from build123d import *

# Parameters (mm, degrees)
F0_W        = 20
F0_H        = 60
F1_DEPTH    = 150
F2_D        = 6
F2_DEPTH    = 50
F2_TIP      = 1.8025818571
F3_SIZE2    = 29.99999
F3_SIZE     = 149.99999
F3_2_SIZE2  = 29.99999
F3_2_SIZE   = 149.99999
F4_T1_DEPTH = 407.0708695577
F4_T3_DEPTH = 407.0708695577


# Not quite as in the source:
# - a fillet or chamfer that OpenCascade refuses, or shapes differently, is made with other operations: its cross-section is extruded or revolved along the edge and cut away or added
# - a fillet or chamfer is up to 0.001 mm smaller than in the source, because OpenCascade refuses the exact size


with BuildPart() as f1:
    # F0 (on Top) → F1 (new body)
    with BuildSketch(Plane.XY):
        Rectangle(F0_W, F0_H)
    extrude(amount=F1_DEPTH)

    # F2
    with Locations(Plane(origin=(0, 0, 0), x_dir=(1, 0, 0), z_dir=(0, 0, -1))):
        with Locations((0, -10), (0, 0), (0, 10)):
            Hole(F2_D / 2, depth=F2_DEPTH)
            with Locations((0, 0, -(F2_DEPTH + F2_TIP / 2))):  # 118° drill point
                Cone(0, F2_D / 2, F2_TIP, mode=Mode.SUBTRACT)

    # F3 (size 150 and 30 in the source; OpenCascade refuses exactly that, so slightly less here)
    f3_edges = [f1.edges().sort_by_distance(p)[0] for p in [
        (0, -30, 150),
    ]]
    f3_side = f1.faces().sort_by_distance((0, -30, 75))[0]
    chamfer(f3_edges, length=F3_SIZE, length2=F3_SIZE2, reference=f3_side)

    # F3#2 (size 150 and 30 in the source; OpenCascade refuses exactly that, so slightly less here)
    f3_2_edges = [f1.edges().sort_by_distance(p)[0] for p in [
        (0, 30, 150),
    ]]
    f3_2_side = f1.faces().sort_by_distance((0, 30, 75))[0]
    chamfer(f3_2_edges, length=F3_2_SIZE, length2=F3_2_SIZE2, reference=f3_2_side)

    # F4: chamfer of 24.5 x 10 on 4 edges, made by hand

    # F4_s2 → F4_t1 (cut)
    with BuildSketch(Plane(origin=(0, -38.5287100353, -192.6436015479), x_dir=(1, 0, 0), z_dir=(0, 0.1961160849, 0.9805806857))):
        Polygon((0, -29.4174225336), (10, -4.9174225336), (10, -29.4174225336), align=None)
        Polygon((-10, -4.9174225336), (0, -29.4174225336), (-10, -29.4174225336), align=None)
    extrude(amount=F4_T1_DEPTH, mode=Mode.SUBTRACT)

    # F4_s4 → F4_t3 (cut)
    with BuildSketch(Plane(origin=(0, 38.5287100353, -192.6436015479), x_dir=(1, 0, 0), z_dir=(0, -0.1961160849, 0.9805806857))):
        Polygon((0, 29.4174225336), (10, 4.9174225336), (10, 29.4174225336), align=None)
        Polygon((-10, 4.9174225336), (0, 29.4174225336), (-10, 29.4174225336), align=None)
    extrude(amount=F4_T3_DEPTH, mode=Mode.SUBTRACT)


solid = f1.part
Source: CAD feature listing. Evaluate the final solid. Frame: model axes, mm. A direction names the side the tool comes from. Give positions to 0.01 mm unless a question says otherwise; leave off trailing zeros. Write each loop counter-clockwise with the first axis right and the second up, starting at its lowest first coordinate (ties: lowest second). Pieces come first, ordered by that corner, then holes. Notation, with made-up numbers: M 85,-13.75 L 127,-13.75 A33 cw 127,24.25 Z; hole C 4,52.25 d9. An arc over 180 degrees is marked long. Return JSON: item names as keys, results as strings. Group by question number.
1) Pin query (flat end, axial travel): P1, Ø1.5, axis at y = 5, z = 83, coming from the +X side; P2, Ø4, axis at y = 8.5, z = 107, coming from the +X side; P3, Ø1.5, axis at y = -1.5, z = 47, coming from the +X side. Return the tip coordinate at first contact, or that it passes through.
2) Cut plane A-A, the plane z = 27.5. Output: boundary loops of the cut face in (x, y), plus the area to 3 significant figures.
3) Cut plane C-C, the plane x = 7.5. Output: boundary loops of the cut face in (y, z), plus the area to 3 significant figures.
4) Material intervals for line 1 along Y through (x, z) = (-1.5, 8); line 2 along X through (y, z) = (11, 19); line 3 along X through (y, z) = (10, 23.5), sorted ascending. Write a range as [from, to].
5) Pull-direction query (Y, two-part tool) for faces 1 (the face through (4, 0, 0)), 2 (the face through (-3.96, 9.03, 55.38)), 3 (the face through (0.24, 0.46, 51.49)), 4 (the face through (0.24, 10.46, 51.49)); classes: pulls with the +Y half, pulls with the -Y half, needs draft (parallel to the pull), parting line crosses it, or undercut.
6) Cut plane D-D, the plane z = 64.5. Output: boundary loops of the cut face in (x, y).
7) Set-up query: faces 5 (the face through (-10, 0, 10)), 6 (the face through (3, -10, 25)). Return all of +Z, -Z, +X, -X, +Y, -Y with unobstructed straight access to the full face (end or side cutting, diameter ignored); none if empty.
8) Cut plane B-B, the plane y = -15.5. Output: boundary loops of the cut face in (x, z), plus the area to 3 significant figures.
Recorded:
{
 "1": {"P1": "stops at x = 3.67", "P2": "stops at x = 0.86", "P3": "stops at x = 7.95"},
 "2": {"outline": "M -9.81,0 L 0,-24.5 L 9.81,0 L 0,24.5 Z; hole C 0,-10 d6; hole C 0,0 d6; hole C 0,10 d6", "area": "396 mm²"},
 "3": {"outline": "M -11.26,0 L 11.26,0 L 0,56.31 Z", "area": "634 mm²"},
 "4": {"line 1": "y = [-24.65, -12.6], [-7.4, -2.6], [2.6, 7.4], [12.6, 24.65]", "line 2": "x = [-6.08, -2.83], [2.83, 6.08]", "line 3": "x = [-6.12, -3], [3, 6.12]"},
 "5": {"face 1": "needs draft", "face 2": "pulls with the +Y half", "face 3": "undercut", "face 4": "undercut"},
 "6": {"outline": "M -6.84,0 L 0,-17.1 L 6.84,0 L 0,17.1 Z"},
 "7": {"face 5": "+Z, -Z, -X, +Y, -Y", "face 6": "-Z"},
 "8": {"outline": "M -5.8,0 L 5.8,0 L 0,72.5 Z", "area": "421 mm²"}
}
